Autodesk Inventor part; units mm, degrees
ref_plane "Work Plane2" through (0, 0, 0) normal (0, 0, 1) x (1, 0, 0)
ref_plane "YZ Plane" through (0, 0, 0) normal (1, 0, 0) x (0, 1, 0)
ref_plane "XZ Plane" through (0, 0, 0) normal (0, 1, 0) x (-1, 0, 0)
ref_plane "Work Plane2" through (0, 0, 0) normal (0, 0, 1) x (1, 0, 0)
sketch "Sketch1" plane through (0, 0, 0) normal (0, 0, 1) x (1, 0, 0)
  line L0 (180, 126) -> (180, 200)
  arc A0 (180, 200) -> (175, 205) centre (175, 200) ccw
  line L1 (175, 205) -> (-174, 205)
  line L2 (-174, -368) -> (-174, 205)
  line L3 (-156, -368) -> (-174, -368)
  arc A1 (-153, -371) -> (-156, -368) centre (-156, -371) ccw
  line L4 (-153, -403) -> (-153, -371)
  arc A2 (-156, -406) -> (-153, -403) centre (-156, -403) ccw
  line L5 (-180, -406) -> (-156, -406)
  line L6 (-180, -406) -> (-180, -480)
  arc A3 (-180, -480) -> (-175, -485) centre (-175, -480) ccw
  line L7 (-175, -485) -> (174, -485)
  line L8 (174, 88) -> (174, -485)
  line L9 (156, 88) -> (174, 88)
  arc A4 (153, 91) -> (156, 88) centre (156, 91) ccw
  line L10 (153, 123) -> (153, 91)
  arc A5 (156, 126) -> (153, 123) centre (156, 123) ccw
  line L11 (180, 126) -> (156, 126)
  circle A6 centre (0, 0) radius 135
  circle A7 centre (82.55, 185) radius 3
  circle A8 centre (-82.55, 185) radius 3
  circle A9 centre (82.55, -460) radius 3
  circle A10 centre (-82.55, -460) radius 3
  line L12 (-149.5, -195) -> (-149.5, -395)
  arc A11 (-149.5, -395) -> (-110, -434.5) centre (-110, -395) ccw
  line L13 (-110, -434.5) -> (110, -434.5)
  arc A12 (110, -434.5) -> (149.5, -395) centre (110, -395) ccw
  line L14 (149.5, -395) -> (149.5, -195)
  arc A13 (149.5, -195) -> (110, -155.5) centre (110, -195) ccw
  line L15 (110, -155.5) -> (-110, -155.5)
  arc A14 (-110, -155.5) -> (-149.5, -195) centre (-110, -195) ccw
  line L16 (40, -245) -> (-40, -245)
  line L17 (-50, -255) -> (-50, -355)
  line L18 (-40, -365) -> (40, -365)
  line L19 (50, -355) -> (50, -255)
  arc A15 (-40, -245) -> (-50, -255) centre (-40, -255) ccw
  arc A16 (50, -255) -> (40, -245) centre (40, -255) ccw
  arc A17 (40, -365) -> (50, -355) centre (40, -355) ccw
  arc A18 (-50, -355) -> (-40, -365) centre (-40, -355) ccw
  point P0 (115, -175)
  point P1 (-50, -365)
  point P2 (-50, -245)
  point P3 (50, -365)
  dimension "d1" = 100
  dimension "d2" = 120
  dimension "d3" = 10
extrude "Extrusion1" add sketch "Sketch1" along normal blind 6.35 contours A14 L15 A13 L14 A12 L13 A11 L12
sketch "Sketch2" plane through (0, 0, 6.35) normal (0, 0, 1) x (1, 0, 0)
  line L0 (180, 126) -> (180, 200)
  arc A0 (180, 200) -> (175, 205) centre (175, 200) ccw
  line L1 (175, 205) -> (-174, 205)
  line L2 (-174, -368) -> (-174, 205)
  line L3 (-156, -368) -> (-174, -368)
  arc A1 (-153, -371) -> (-156, -368) centre (-156, -371) ccw
  line L4 (-153, -403) -> (-153, -371)
  arc A2 (-156, -406) -> (-153, -403) centre (-156, -403) ccw
  line L5 (-180, -406) -> (-156, -406)
  line L6 (-180, -406) -> (-180, -480)
  arc A3 (-180, -480) -> (-175, -485) centre (-175, -480) ccw
  line L7 (-175, -485) -> (174, -485)
  line L8 (174, 88) -> (174, -485)
  line L9 (156, 88) -> (174, 88)
  arc A4 (153, 91) -> (156, 88) centre (156, 91) ccw
  line L10 (153, 123) -> (153, 91)
  arc A5 (156, 126) -> (153, 123) centre (156, 123) ccw
  line L11 (180, 126) -> (156, 126)
  circle A6 centre (0, 0) radius 135
  circle A7 centre (-140, -217) radius 2
  circle A8 centre (-140, -269) radius 2
  circle A9 centre (-140, -321) radius 2
  circle A10 centre (-140, -373) radius 2
  circle A11 centre (-84, -425) radius 2
  circle A12 centre (-28, -425) radius 2
  circle A13 centre (28, -425) radius 2
  circle A14 centre (84, -425) radius 2
  circle A15 centre (140, -373) radius 2
  circle A16 centre (140, -321) radius 2
  circle A17 centre (140, -269) radius 2
  circle A18 centre (140, -217) radius 2
  circle A19 centre (84, -165) radius 2
  circle A20 centre (28, -165) radius 2
  circle A21 centre (-28, -165) radius 2
  circle A22 centre (-84, -165) radius 2
  line L12 (-130, -190) -> (-130, -400)
  arc A23 (-115, -175) -> (-130, -190) centre (-115, -190) ccw
  line L13 (115, -175) -> (-115, -175)
  arc A24 (130, -190) -> (115, -175) centre (115, -190) ccw
  line L14 (130, -400) -> (130, -190)
  arc A25 (115, -415) -> (130, -400) centre (115, -400) ccw
  line L15 (-115, -415) -> (115, -415)
  arc A26 (-130, -400) -> (-115, -415) centre (-115, -400) ccw
  circle A27 centre (82.55, 185) radius 3
  circle A28 centre (-82.55, 185) radius 3
  circle A29 centre (82.55, -460) radius 3
  circle A30 centre (-82.55, -460) radius 3
hole "Hole1" at (-140, -217, 6.35) at (-84, -165, 6.35) at (-28, -165, 6.35) at (28, -165, 6.35) at (84, -165, 6.35) at (-140, -269, 6.35) at (-140, -321, 6.35) at (-140, -373, 6.35) at (-84, -425, 6.35) at (-28, -425, 6.35) at (28, -425, 6.35) at (84, -425, 6.35) at (140, -373, 6.35) at (140, -321, 6.35) at (140, -269, 6.35) at (140, -217, 6.35) direction (0, 0, -1) diameter 5.5 end through all counterbore diameter 12.24 counterbore depth 2
sketch "Sketch3" plane through (0, 0, 6.35) normal (0, 0, 1) x (1, 0, 0)
  point P0 (0, 0)
  point P1 (-65, -305)
  point P2 (-65, -260)
  point P3 (-65, -350)
  point P4 (65, -305)
  point P5 (65, -260)
  point P6 (65, -350)
  point P7 (-20, -230)
  point P8 (20, -230)
  point P9 (-20, -380)
  point P10 (20, -380)
  dimension "d18" = 45
  dimension "d19" = 45
  dimension "d22" = 45
  dimension "d23" = 45
hole "Hole2" at (-65, -305, 6.35) at (-65, -260, 6.35) at (-65, -350, 6.35) at (65, -305, 6.35) at (65, -260, 6.35) at (65, -350, 6.35) at (-20, -230, 6.35) at (20, -230, 6.35) at (-20, -380, 6.35) at (20, -380, 6.35) direction (0, 0, -1) diameter 3.4587 depth 10.8 tip angle 118
properties part number "Reducer Plate" material "Aluminum 6061"
For this review, take the finished solid that the model builds, in its own axes (mm). A direction names the side the tool comes from. Give positions to 0.01 mm unless a question says otherwise; leave off trailing zeros. Order: outer loops, then holes, each group sorted by start corner. A loop starts at its lowest first (then second) coordinate and runs counter-clockwise, first axis right, second up. Notation, with made-up numbers: (87.25, 37.5) - (134.25, 37.5) arc R24 ccw to (134.25, 72.5) - close; hole circle Ø7 at (69.5, -22.75). An arc over 180 degrees is marked (long way). Answer as a JSON object with one key per item and string values. Group by question number.
Item 1: Take a section at B-B on z = 2.75. Give the number of separate pieces and of enclosed holes in the cut face, and give its area (3 significant figures).
Item 2: Draft analysis for pull direction X (two halves, no side actions). For faces 1 (the cylindrical face through (139.731, -366.886, 5.336)), 2 (the cylindrical face through (-138.24, -167.38, 3.13)), 3 (the cylindrical face through (138.24, -422.62, 3.13)), 4 (the cylindrical face through (-140.269, -366.886, 5.336)), state which applies: pulls with the +X half, pulls with the -X half, needs draft (parallel to the pull), parting line crosses it, or undercut.
Item 3: Take a section at A-A on y = -297.5. Give the boundary of the cut face in (x, z), and give its area (3 significant figures).
Item 4: Wall thickness on line 1 along X through (y, z) = (-217, 0.95); line 2 along Y through (x, z) = (-28, 2.2); line 3 along Y through (x, z) = (-84, 5.6): over which ranges is each line inside the solid? List them lowest first.
Item 5: Machinability: for faces 5 (the flat face through (-2, -434.5, 3)), 6 (the cylindrical face through (139.731, -262.886, 5.336)), 7 (the flat face through (-50, -304, 3)), which of the approach directions +Z, -Z, +X, -X, +Y, -Y give a long, thin tool a straight path to every point of the face, cutting with its end or side? Answer none if there is none.
Item 6: Clearance check with flat-ended pins moving along their axes: pin 1 Ø2 at (x, y) = (-20, -380) entering from +Z; pin 2 Ø10 at (x, y) = (31, -427.5) entering from +Z; pin 3 Ø6 at (x, y) = (-139.5, -319) entering from +Z. State where each tip first meets the part, or that it passes through.
Reported:
{
 "1": {"separate pieces": "1", "enclosed holes": "27", "area": "69,700 mm^2"},
 "2": {"face 1": "undercut", "face 2": "pulls with the -X half", "face 3": "pulls with the +X half", "face 4": "undercut"},
 "3": {"outline": "(-149.5, 0) - (-50, 0) - (-50, 6.35) - (-149.5, 6.35) - close; (50, 0) - (149.5, 0) - (149.5, 6.35) - (50, 6.35) - close", "area": "1,260 mm^2"},
 "4": {"line 1": "-149.5 to -142.75, -137.25 to 137.25, 142.75 to 149.5", "line 2": "-434.5 to -427.75, -422.25 to -365, -245 to -167.75, -162.25 to -155.5", "line 3": "-434.5 to -431.12, -418.88 to -171.12, -158.88 to -155.5"},
 "5": {"face 5": "+Z, -Z, +X, -X, -Y", "face 6": "+Z", "face 7": "+Z, -Z"},
 "6": {"pin 1": "through", "pin 2": "z = 6.35", "pin 3": "z = 4.35"}
}
